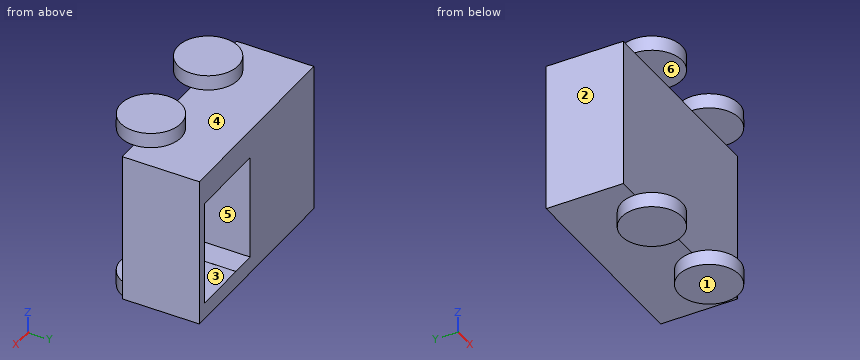
```python
from build123d import *

# Parameters (mm, degrees)
SKETCH7_W           = 20
SKETCH7_H           = 7.663039205
BOSS_EXTRUDE2_DEPTH = 15
SKETCH8_W           = 5.5
SKETCH8_H           = 10.5
CUT_EXTRUDE3_DEPTH  = 7
SKETCH9_R           = 3
BOSS_EXTRUDE4_DEPTH = 1.5
SKETCH11_R          = 3
BOSS_EXTRUDE6_DEPTH = 1.5
SKETCH12_R          = 3
BOSS_EXTRUDE7_DEPTH = 1.5
SKETCH13_W          = 2.5
SKETCH13_H          = 10.495878043
CUT_EXTRUDE4_DEPTH  = 7


with BuildPart() as part:
    # Sketch7 → Boss-Extrude2 (new body)
    with BuildSketch(Plane.XY):
        with Locations((10, -3.831519603)):
            Rectangle(SKETCH7_W, SKETCH7_H)
    extrude(amount=BOSS_EXTRUDE2_DEPTH)

    # Sketch8 → Cut-Extrude3 (cut)
    with BuildSketch(Plane(origin=(0, 0, 0), x_dir=(1, 0, 0), z_dir=(0, 1, 0))):
        with Locations((16.367319257, -6.904304489)):
            Rectangle(SKETCH8_W, SKETCH8_H)
    extrude(amount=-CUT_EXTRUDE3_DEPTH, mode=Mode.SUBTRACT)

    # Sketch9 → Boss-Extrude4 (add)
    with BuildSketch(Plane.XY.offset(15)):
        with Locations((15, -7.663039205)):
            Circle(SKETCH9_R)
    extrude(amount=BOSS_EXTRUDE4_DEPTH)

    # Sketch11 → Boss-Extrude6 (add)
    with BuildSketch(Plane.XY.offset(15)):
        with Locations((5, -7.663039205)):
            Circle(SKETCH11_R)
    extrude(amount=BOSS_EXTRUDE6_DEPTH)

    # Sketch12 → Boss-Extrude7 (add)
    with BuildSketch(Plane(origin=(0, 0, 0), x_dir=(-1, 0, 0), z_dir=(0, 0, -1))):
        with Locations((-15, -7.663039205)):
            Circle(SKETCH12_R)
        with Locations((-5, -7.663039205)):
            Circle(SKETCH12_R)
    extrude(amount=BOSS_EXTRUDE7_DEPTH)

    # Sketch13 → Cut-Extrude4 (cut)
    with BuildSketch(Plane(origin=(0, 0, 0), x_dir=(1, 0, 0), z_dir=(0, 1, 0))):
        with Locations((12.367319257, -6.906365468)):
            Rectangle(SKETCH13_W, SKETCH13_H)
    extrude(amount=-CUT_EXTRUDE4_DEPTH, mode=Mode.SUBTRACT)


solid = part.part
```
Check sheet for the modelled part. Datum: model origin and axes. Units: mm. Face numbers are marked on the shaded views. A direction names the side the tool comes from. Give positions to 0.01 mm unless a question says otherwise; leave off trailing zeros. Write each loop counter-clockwise with the first axis right and the second up, starting at its lowest first coordinate (ties: lowest second). Pieces come first, ordered by that corner, then holes.
Item 1: Cross-section at D-D (x = 15). Enter the section's corners in (y, z).
Item 2: Cross-section at C-C (z = 7.5). Enter the section's corners in (x, y).
Item 3: Scan lines: L1, parallel to Z at x = 11.25, y = -3; L2, parallel to Z at x = 13.75, y = -5; L3, parallel to X at y = -3, z = 1.75. Record each from-to range of solid material in increasing order.
Item 4: Gauge pin test, flat ends, axial feed: pin 1 (1.2 mm diameter, centred on x = 12, y = -3, fed in from +Z); pin 2 (6 mm diameter, centred on x = 9.5, y = -2, fed in from -Z); pin 3 (1 mm diameter, centred on y = -9, z = 7, fed in from +X). Record the tip position at first contact, or that the pin passes through.
Item 5: Cross-section at A-A (y = -9.25). Enter the section's corners in (x, z).
Item 6: Draft check along X on the marked faces 1, 2 and 3. Enter one of: released by +X, released by -X, zero draft, split by the parting line, or undercut.
Item 7: Access from +Z, -Z, +X, -X, +Y, -Y to the whole of each face (thin tool, end or side, straight path). Record for the marked faces 4, 5 and 6.
Report:
1. outline: (-10.66, -1.5) - (-4.66, -1.5) - (-4.66, 0) - (0, 0) - (0, 1.65) - (-7, 1.65) - (-7, 12.15) - (0, 12.15) - (0, 15) - (-4.66, 15) - (-4.66, 16.5) - (-10.66, 16.5) - (-10.66, 15) - (-7.66, 15) - (-7.66, 0) - (-10.66, 0) - close
2. outline: (0, -7.66) - (20, -7.66) - (20, 0) - (19.12, 0) - (19.12, -7) - (11.12, -7) - (11.12, 0) - (0, 0) - close
3. L1: z = 0 to 1.66, 12.15 to 15
3. L2: z = -1.5 to 1.65, 12.15 to 16.5
3. L3: x = 0 to 11.12, 19.12 to 20
4. pin 1: stops at z = 15
4. pin 2: stops at z = 0
4. pin 3: passes through
5. outline: (2.45, -1.5) - (7.55, -1.5) - (7.55, 0) - (2.45, 0) - close; (2.45, 15) - (7.55, 15) - (7.55, 16.5) - (2.45, 16.5) - close; (12.45, -1.5) - (17.55, -1.5) - (17.55, 0) - (12.45, 0) - close; (12.45, 15) - (17.55, 15) - (17.55, 16.5) - (12.45, 16.5) - close
6. face 1: zero draft
6. face 2: released by -X
6. face 3: undercut
7. face 4: +Z, +Y
7. face 5: +Y
7. face 6: +X, -X, -Y
